from build123d import *

# Parameters (mm, degrees)
F0_W     = 90
F0_H     = 70
F1_DEPTH = 5
F2_W     = 5
F2_H     = 70
F3_DEPTH = 110
F4_W     = 40
F4_H     = 5
F5_DEPTH = 65
F6_W     = 40
F6_H     = 5
F7_DEPTH = 80
F8_SIZE  = 4.99999


# Not quite as in the source:
# - a fillet or chamfer is up to 0.001 mm smaller than in the source, because OpenCascade refuses the exact size


with BuildPart() as f1:
    # F0 (on Right) → F1 (new body)
    with BuildSketch(Plane.YZ):
        Rectangle(F0_W, F0_H)
    extrude(amount=-F1_DEPTH)

    # F2 (on face) → F3 (join)
    with BuildSketch(Plane(origin=(-5, 0, 0), x_dir=(0, -1, 0), z_dir=(-1, 0, 0))):
        with Locations((-42.5, 0)):
            Rectangle(F2_W, F2_H)
        with Locations((42.5, 0)):
            Rectangle(F2_W, F2_H)
    extrude(amount=F3_DEPTH)

    # F4 (on face) → F5 (join)
    with BuildSketch(Plane(origin=(0, 0, -35), x_dir=(1, 0, 0), z_dir=(0, 0, -1))):
        with Locations((-95, 42.5)):
            Rectangle(F4_W, F4_H)
        with Locations((-95, -42.5)):
            Rectangle(F4_W, F4_H)
    extrude(amount=F5_DEPTH)

    # F6 (on face) → F7 (join, through all)
    with BuildSketch(Plane(origin=(0, -40, 0), x_dir=(-1, 0, 0), z_dir=(0, 1, 0))):
        with Locations((95, -97.5)):
            Rectangle(F6_W, F6_H)
    extrude(amount=F7_DEPTH)

    # F8 (size 5 in the source; OpenCascade refuses exactly that, so slightly less here)
    f8_edges = [f1.edges().sort_by_distance(p)[0] for p in [
        (0, 0, 35),
        (-115, 42.5, 35),
        (-115, -42.5, 35),
        (-95, -45, -100),
        (-95, -40, -95),
        (-95, 40, -95),
        (-95, 45, -100),
    ]]
    chamfer(f8_edges, length=F8_SIZE)


solid = f1.part
Can you work these out from the model? Positions are in its coordinate system, mm. A direction names the side the tool comes from. Coordinates: 2 decimals unless noted, no trailing zeros. Loops run counter-clockwise (first coordinate to the right, second up) from the corner with the lowest first, then second, coordinate; pieces in that order, holes last. Notation, with made-up numbers: (89.25, -17.5) - (141.25, -17.5) arc R30 ccw to (141.25, 19.5) - close; hole circle Ø8 at (60, -21.5). An arc over 180 degrees is marked (long way). Put each result on its own line as item: value. Start each with the question number.
Item 1: If I drill on line 1 along Y through (x, z) = (-100, -45); line 2 along Z through (x, y) = (-57.5, 41); line 3 along Z through (x, y) = (-86.5, -27.5), over which ranges is the centre line in solid material (lowest first)?
Item 2: For pin 1 (21 mm diameter, centred on y = -11, z = -11.5, fed in from -X), with a flat end and sliding along its axis, tell me the tip position at first contact or that it passes through.
Item 3: Suppose I cut it at B-B (x = -34). Please give me the cut outline in (y, z).
Item 4: If we mould it in two halves opening along Y, with no side actions, what happens to faces 6 (the face through (-95, 38, -92)), 7 (the face through (-71, -45, -15)), 8 (the face through (-95, -1, -100))? For each: +Y half, -Y half, draft (parallel to the pull), parting line (faces both ways), or undercut.
Item 5: Suppose I cut it at A-A (z = -77). Please give me the cut outline in (x, y).
Item 6: Suppose I cut it at D-D (x = -90). Please give me the cut outline in (y, z), and give its area (3 significant figures).
Item 7: Which directions (+Z, -Z, +X, -X, +Y, -Y) give clear straight access to the entire face, cutting with the end or side of a thin tool? Please do faces 1 (the face through (-75, -7, -97)), 2 (the face through (-2, -1, 32)), 3 (the face through (-95, 0, -95)), 4 (the face through (-73, -40, -13)), 5 (the face through (-5, -1, 0)).
Here are the results:
1. line 1: -45 to -40, 40 to 45
1. line 2: -35 to 35
1. line 3: -100 to -95
2. pin 1: x = -5
3. outline: (-45, -35) - (-40, -35) - (-40, 35) - (-45, 35) - close; (40, -35) - (45, -35) - (45, 35) - (40, 35) - close
4. face 6: undercut
4. face 7: -Y half
4. face 8: draft
5. outline: (-115, -45) - (-75, -45) - (-75, -40) - (-115, -40) - close; (-115, 40) - (-75, 40) - (-75, 45) - (-115, 45) - close
6. outline: (-45, -95) - (-40, -100) - (40, -100) - (45, -95) - (45, 35) - (40, 35) - (40, -90) - (35, -95) - (-35, -95) - (-40, -90) - (-40, 35) - (-45, 35) - close
6. area: 1,750 mm²
7. face 1: -Z, +X, +Y, -Y
7. face 2: +Z, +X, +Y, -Y
7. face 3: +Z, +X, -X
7. face 4: +Z, -X
7. face 5: +Z, -Z, -X
